Geometry check sheet. Reference: drawing and pictorial views, mm from the part's lowest x, y, z. Round coordinates to 2 decimals unless told otherwise and drop trailing zeros. Order: outer loops, then holes, each group sorted by start corner. A loop starts at its lowest first (then second) coordinate and runs counter-clockwise, first axis right, second up.
(1) Sectioned sample at B-B (y = 55). Record the boundary of the cut face in (x, z), plus the area to 3 significant figures.
(2) Material ranges on line 1 along X through (y, z) = (8, 1.1); line 2 along Y through (x, z) = (5, 2.15); line 3 along Y through (x, z) = (29, 1.1), recorded low to high.
(3) Sectioned sample at C-C (z = 1.05). Record the boundary of the cut face in (x, y).
(4) Sectioned sample at A-A (x = 17.5). Record the boundary of the cut face in (y, z), plus the area to 3 significant figures.
(5) Sectioned sample at D-D (x = 6). Record the boundary of the cut face in (y, z), plus the area to 3 significant figures.
(6) Go/stop test with a flat-tipped pin: pin 1 (2 mm diameter, centred on x = 6, y = 61.75, fed in from +Z). Record where the tip stops, or that it passes through.
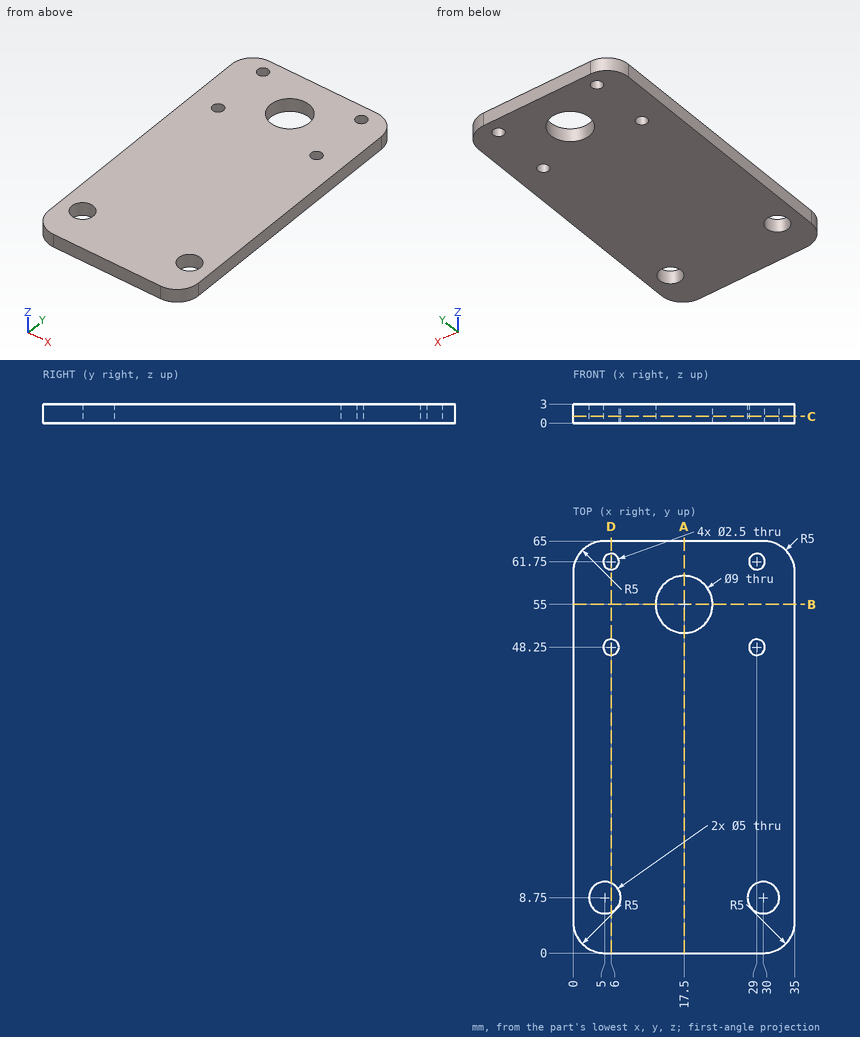
Answer below:
1. outline: (0, 0) - (13, 0) - (13, 3) - (0, 3) - close; (22, 0) - (35, 0) - (35, 3) - (22, 3) - close
1. area: 78.0 mm2
2. line 1: x = 0 to 2.62, 7.38 to 27.62, 32.38 to 35
2. line 2: y = 0 to 6.25, 11.25 to 47.5, 49 to 61, 62.5 to 65
2. line 3: y = 0 to 6.46, 11.04 to 47, 49.5 to 60.5, 63 to 65
3. outline: (0, 5) arc R5 ccw to (5, 0) - (30, 0) arc R5 ccw to (35, 5) - (35, 60) arc R5 ccw to (30, 65) - (5, 65) arc R5 ccw to (0, 60) - close; hole circle Ø5 at (5, 8.75); hole circle Ø2.5 at (6, 48.25); hole circle Ø2.5 at (6, 61.75); hole circle Ø9 at (17.5, 55); hole circle Ø5 at (30, 8.75); hole circle Ø2.5 at (29, 48.25); hole circle Ø2.5 at (29, 61.75)
4. outline: (0, 0) - (50.5, 0) - (50.5, 3) - (0, 3) - close; (59.5, 0) - (65, 0) - (65, 3) - (59.5, 3) - close
4. area: 168 mm2
5. outline: (0, 0) - (6.46, 0) - (6.46, 3) - (0, 3) - close; (11.04, 0) - (47, 0) - (47, 3) - (11.04, 3) - close; (49.5, 0) - (60.5, 0) - (60.5, 3) - (49.5, 3) - close; (63, 0) - (65, 0) - (65, 3) - (63, 3) - close
5. area: 166 mm2
6. pin 1: passes through
